```python
from build123d import *

# Parameters (mm, degrees)
SKETCH1_R           = 3
BOSS_EXTRUDE1_DEPTH = 4
SKETCH2_R           = 4.763139721
SKETCH2_R_2         = 3
BOSS_EXTRUDE2_DEPTH = 2


with BuildPart() as part:
    # Sketch1 → Boss-Extrude1 (new body)
    with BuildSketch(Plane(origin=(0, 0, 0), x_dir=(1, 0, 0), z_dir=(0, 1, 0))):
        Polygon((0, 5.5), (-4.763139721, 2.75), (-4.763139721, -2.75), (0, -5.5), (4.763139721, -2.75), (4.763139721, 2.75), align=None)
        with Locations(Location((0, 0, 0), (0, 0, 270))):
            Circle(SKETCH1_R, mode=Mode.SUBTRACT)
    extrude(amount=BOSS_EXTRUDE1_DEPTH)

    # Sketch2 → Boss-Extrude2 (add)
    with BuildSketch(Plane(origin=(0, 4, 0), x_dir=(1, 0, 0), z_dir=(0, 1, 0))):
        with Locations(Location((0, 0, 0), (0, 0, 60))):
            Circle(SKETCH2_R)
        with Locations(Location((0, 0, 0), (0, 0, 270))):
            Circle(SKETCH2_R_2, mode=Mode.SUBTRACT)
    extrude(amount=BOSS_EXTRUDE2_DEPTH)


solid = part.part
```
Could you check a few things on this model? Use its own coordinates, in mm. A direction names the side the tool comes from. Coordinates: 2 decimals unless noted, no trailing zeros. Order: outer loops, then holes, each group sorted by start corner. A loop starts at its lowest first (then second) coordinate and runs counter-clockwise, first axis right, second up. Notation, with made-up numbers: M 64,-4 L 104,-4 A21 cw 104,2 Z; hole C 46.5,63.25 d9. An arc over 180 degrees is marked long. Use a Markdown table: item, result. Add a question column.
Q1. Which directions (+Z, -Z, +X, -X, +Y, -Y) give clear straight access to the entire face, cutting with the end or side of a thin tool? Please do faces 5 (the flat face through (-4.3, 4, -2.4)), 6 (the flat face through (-4, 4, 3)), 7 (the flat face through (0, 4, 5)).
Q2. We'd pull the mould along Z, two halves only. Please class faces 1 (the cylindrical face through (3.78, 4.99, -2.9)), 2 (the flat face through (2.1, 0, 2.4)), 3 (the flat face through (2.348, 1.972, 4.144)), 4 (the cylindrical face through (0.9, 2.96, 2.86)): pulls with the +Z half, pulls with the -Z half, needs draft (parallel to the pull), parting line crosses it, or undercut.
Q3. I want a section at B-B on z = -2.5. List the corners of the cut face in (x, y) for me.
Q4. I want a section at D-D on x = 4. List the corners of the cut face in (y, z) for me, then the cut area to 3 significant figures.
Q5. If I drill on L1, parallel to X at y = 3.6, z = 0; L2, parallel to Z at x = 1.75, y = 2.45; L3, parallel to X at y = 1.05, z = -0.75, over which ranges is the centre line in solid material (lowest first)?
Q6. I want a section at A-A on y = 1.8. List the corners of the cut face in (x, z) for me.
Q7. I want a section at C-C on x = 1. List the corners of the cut face in (y, z) for me.
Checked values:
| question | item | result |
|---|---|---|
| 1 | face 5 | -Z, -X, +Y |
| 1 | face 6 | +Z, -X, +Y |
| 1 | face 7 | +Z, +Y |
| 2 | face 1 | parting line crosses it |
| 2 | face 2 | needs draft |
| 2 | face 3 | pulls with the +Z half |
| 2 | face 4 | undercut |
| 3 | outline | M -4.76,0 L -1.66,0 L -1.66,6 L -4.05,6 L -4.05,4 L -4.76,4 Z; M 1.66,0 L 4.76,0 L 4.76,4 L 4.05,4 L 4.05,6 L 1.66,6 Z |
| 4 | outline | M 0,-3.19 L 4,-3.19 L 4,-2.59 L 6,-2.59 L 6,2.59 L 4,2.59 L 4,3.19 L 0,3.19 Z |
| 4 | area | 35.9 mm² |
| 5 | L1 | -4.76 to -3, 3 to 4.76 |
| 5 | L2 | -4.49 to -2.44, 2.44 to 4.49 |
| 5 | L3 | -4.76 to -2.9, 2.9 to 4.76 |
| 6 | outline | M -4.76,-2.75 L 0,-5.5 L 4.76,-2.75 L 4.76,2.75 L 0,5.5 L -4.76,2.75 Z; hole C 0,0 d6 |
| 7 | outline | M 0,-4.92 L 4,-4.92 L 4,-4.66 L 6,-4.66 L 6,-2.83 L 0,-2.83 Z; M 0,2.83 L 6,2.83 L 6,4.66 L 4,4.66 L 4,4.92 L 0,4.92 Z |
